Build history of the part. All positions in model axes, mm. A direction names the side the tool comes from. Coordinates: 2 decimals unless noted, no trailing zeros. Write each loop counter-clockwise with the first axis right and the second up, starting at its lowest first coordinate (ties: lowest second). Pieces come first, ordered by that corner, then holes.
```python
from build123d import *

# Parameters (mm, degrees)
SKETCH1_W           = 50
SKETCH1_H           = 110
BOSS_EXTRUDE1_DEPTH = 2
SKETCH2_W           = 50
SKETCH2_H           = 110
SKETCH2_W_2         = 46
SKETCH2_H_2         = 106
BOSS_EXTRUDE3_DEPTH = 11
SKETCH3_R           = 1.2
BOSS_EXTRUDE4_DEPTH = 11
SKETCH4_W           = 52
SKETCH4_H           = 112
SKETCH4_W_2         = 50
SKETCH4_H_2         = 110
EXTRUDE_THIN1_DEPTH = 13
FILLET2_R           = 2
EXTRUDE_THIN3_DEPTH = 3
SKETCH6_R           = 1.8
BOSS_EXTRUDE5_DEPTH = 2.8
SKETCH8_W           = 8
SKETCH8_H           = 3.6
CUT_EXTRUDE2_DEPTH  = 12.8
SKETCH11_W          = 13.1
SKETCH11_H          = 5.8
CUT_EXTRUDE5_DEPTH  = 3


with BuildPart() as part:
    # Sketch1 → Boss-Extrude1 (new body)
    with BuildSketch(Plane(origin=(0, 0, 0), x_dir=(1, 0, 0), z_dir=(0, 1, 0))):
        with Locations((-52.022587269, -1.919917864)):
            Rectangle(SKETCH1_W, SKETCH1_H)
    extrude(amount=BOSS_EXTRUDE1_DEPTH)

    # Sketch2 → Boss-Extrude3 (add)
    with BuildSketch(Plane(origin=(0, 2, 0), x_dir=(1, 0, 0), z_dir=(0, 1, 0))):
        with Locations((-52.022587269, -1.919917864)):
            Rectangle(SKETCH2_W, SKETCH2_H)
        with Locations((-52.022587269, -1.919917864)):
            Rectangle(SKETCH2_W_2, SKETCH2_H_2, mode=Mode.SUBTRACT)
    extrude(amount=BOSS_EXTRUDE3_DEPTH)

    # Sketch3 → Boss-Extrude4 (add)
    with BuildSketch(Plane(origin=(0, 2, 0), x_dir=(1, 0, 0), z_dir=(0, 1, 0))):
        with Locations((-31.022587269, 42.380082136)):
            Circle(SKETCH3_R)
        with Locations((-31.022587269, -52.919917864)):
            Circle(SKETCH3_R)
        with Locations((-56.322587269, 42.380082136)):
            Circle(SKETCH3_R)
        with Locations((-56.322587269, -52.919917864)):
            Circle(SKETCH3_R)
    extrude(amount=BOSS_EXTRUDE4_DEPTH)

    # Sketch4 → Extrude-Thin1 (add)
    with BuildSketch(Plane(origin=(0, 13, 0), x_dir=(1, 0, 0), z_dir=(0, 1, 0))):
        with Locations((-52.022587269, -1.919917864)):
            Rectangle(SKETCH4_W, SKETCH4_H)
        with Locations((-52.022587269, -1.919917864)):
            Rectangle(SKETCH4_W_2, SKETCH4_H_2, mode=Mode.SUBTRACT)
    extrude(amount=-EXTRUDE_THIN1_DEPTH)

    # Fillet2
    fillet2_edges = [part.edges().sort_by_distance(p)[0] for p in [
        (-26.022587269, 6.5, -54.080082136),
        (-26.022587269, 6.5, 57.919917864),
        (-78.022587269, 6.5, 57.919917864),
        (-78.022587269, 6.5, -54.080082136),
    ]]
    fillet(fillet2_edges, radius=FILLET2_R)

    # Sketch5 → Extrude-Thin3 (add)
    with BuildSketch(Plane(origin=(0, 13, 0), x_dir=(1, 0, 0), z_dir=(0, 1, 0))):
        with BuildLine():
            Line((-28.022587269, 54.080082136), (-76.022587269, 54.080082136))
            ThreePointArc((-76.022587269, 54.080082136), (-77.436800831, 53.494295698), (-78.022587269, 52.080082136))
            Line((-78.022587269, 52.080082136), (-78.022587269, -55.919917864))
            ThreePointArc((-78.022587269, -55.919917864), (-77.436800831, -57.334131427), (-76.022587269, -57.919917864))
            Line((-76.022587269, -57.919917864), (-28.022587269, -57.919917864))
            ThreePointArc((-28.022587269, -57.919917864), (-26.608373707, -57.334131427), (-26.022587269, -55.919917864))
            Line((-26.022587269, -55.919917864), (-26.022587269, 52.080082136))
            ThreePointArc((-26.022587269, 52.080082136), (-26.608373707, 53.494295698), (-28.022587269, 54.080082136))
        make_face()
        with BuildLine():
            Line((-28.022587269, 52.880082136), (-76.022587269, 52.880082136))
            ThreePointArc((-76.022587269, 52.880082136), (-76.588272694, 52.64576756), (-76.822587269, 52.080082136))
            Line((-76.822587269, 52.080082136), (-76.822587269, -55.919917864))
            ThreePointArc((-76.822587269, -55.919917864), (-76.588272694, -56.485603289), (-76.022587269, -56.719917864))
            Line((-76.022587269, -56.719917864), (-28.022587269, -56.719917864))
            ThreePointArc((-28.022587269, -56.719917864), (-27.456901844, -56.485603289), (-27.222587269, -55.919917864))
            Line((-27.222587269, -55.919917864), (-27.222587269, 52.080082136))
            ThreePointArc((-27.222587269, 52.080082136), (-27.456901844, 52.64576756), (-28.022587269, 52.880082136))
        make_face(mode=Mode.SUBTRACT)
    extrude(amount=EXTRUDE_THIN3_DEPTH)

    # Sketch6 → Boss-Extrude5 (add)
    with BuildSketch(Plane(origin=(0, 2, 0), x_dir=(1, 0, 0), z_dir=(0, 1, 0))):
        with Locations((-56.322587269, -52.919917864)):
            Circle(SKETCH6_R)
        with Locations((-31.022587269, -52.919917864)):
            Circle(SKETCH6_R)
        with Locations((-56.322587269, 42.380082136)):
            Circle(SKETCH6_R)
        with Locations((-31.022587269, 42.380082136)):
            Circle(SKETCH6_R)
    extrude(amount=BOSS_EXTRUDE5_DEPTH)

    # Sketch8 → Cut-Extrude2 (cut)
    with BuildSketch(Plane(origin=(-26.022587269, 0, 0), x_dir=(0, 0, -1), z_dir=(1, 0, 0))):
        with Locations((-44.619917864, 3.8)):
            Rectangle(SKETCH8_W, SKETCH8_H)
    extrude(amount=-CUT_EXTRUDE2_DEPTH, mode=Mode.SUBTRACT)

    # Sketch11 → Cut-Extrude5 (cut)
    with BuildSketch(Plane.ZY.offset(78.022587269)):
        with Locations((-43.530082136, 4.9)):
            Rectangle(SKETCH11_W, SKETCH11_H)
    extrude(amount=-CUT_EXTRUDE5_DEPTH, mode=Mode.SUBTRACT)


solid = part.part
```
1. Flat gauge pins, fed straight in: pin 1 (1.9 mm diameter, centred on x = -31.5, z = 52.5, fed in from +Y); pin 2 (2 mm diameter, centred on x = -45, z = 33, fed in from +Y). Where does each tip first touch, or does it go through?
Computed values:
pin 1: stops at y = 13
pin 2: stops at y = 2
2. Mould opens along Y. For faces 6 (the face through (-26.023, 8, 3)), 7 (the face through (-31, 13, -42)), 8 (the face through (-77, 5, -36.98)) say: +Y half, -Y half, draft (parallel to the pull), parting line (faces both ways), or undercut.
Computed values:
face 6: draft
face 7: +Y half
face 8: undercut
3. Saw through at A-A on y = 15. List the corners of the cut face in (x, z).
Computed values:
outline: (-78.02, -52.08) arc R2 ccw to (-76.02, -54.08) - (-28.02, -54.08) arc R2 ccw to (-26.02, -52.08) - (-26.02, 55.92) arc R2 ccw to (-28.02, 57.92) - (-76.02, 57.92) arc R2 ccw to (-78.02, 55.92) - close; hole (-76.82, -52.08) arc R0.8 ccw to (-76.02, -52.88) - (-28.02, -52.88) arc R0.8 ccw to (-27.22, -52.08) - (-27.22, 55.92) arc R0.8 ccw to (-28.02, 56.72) - (-76.02, 56.72) arc R0.8 ccw to (-76.82, 55.92) - close
4. Saw through at C-C on x = -70.5. List the corners of the cut face in (y, z).
Computed values:
outline: (0, -54.08) - (16, -54.08) - (16, -52.88) - (13, -52.88) - (13, -51.08) - (2, -51.08) - (2, 54.92) - (13, 54.92) - (13, 56.72) - (16, 56.72) - (16, 57.92) - (0, 57.92) - close
5. 3-axis set-ups, long thin cutter, end or side, ignore diameter. For faces 1 (the face through (-29.023, 7, 3)), 2 (the face through (-52, 0, 1)), 3 (the face through (-77, 16, 2)), 4 (the face through (-77, 7.8, -44)), 5 (the face through (-28, 5.6, 45)): which of +Z, -Z, +X, -X, +Y, -Y reach the whole face in a straight line?
Computed values:
face 1: +Y
face 2: +Z, -Z, +X, -X, -Y
face 3: +Z, -Z, +X, -X, +Y
face 4: -X
face 5: +X
6. Saw through at D-D on y = 6.75. List the corners of the cut face in (x, z), plus the area to 3 significant figures.
Computed values:
outline: (-78.02, -52.08) arc R2 ccw to (-76.02, -54.08) - (-28.02, -54.08) arc R2 ccw to (-26.02, -52.08) - (-26.02, 55.92) arc R2 ccw to (-28.02, 57.92) - (-76.02, 57.92) arc R2 ccw to (-78.02, 55.92) - (-78.02, -36.98) - (-75.02, -36.98) - (-75.02, 54.92) - (-29.02, 54.92) - (-29.02, -51.08) - (-75.02, -51.08) - (-75.02, -50.08) - (-78.02, -50.08) - close; circle Ø2.4 at (-56.32, -42.38); circle Ø2.4 at (-56.32, 52.92); circle Ø2.4 at (-31.02, -42.38); circle Ø2.4 at (-31.02, 52.92)
area: 923 mm2
7. Saw through at B-B on z = -16.5. List the corners of the cut face in (x, y), plus the area to 3 significant figures.
Computed values:
outline: (-78.02, 0) - (-26.02, 0) - (-26.02, 16) - (-27.22, 16) - (-27.22, 13) - (-29.02, 13) - (-29.02, 2) - (-75.02, 2) - (-75.02, 13) - (-76.82, 13) - (-76.82, 16) - (-78.02, 16) - close
area: 177 mm2
8. Probe line 1 along Z through (x, y) = (-44.5, 15.75); line 2 along Z through (x, y) = (-35, 10.25); line 3 along X through (y, z) = (10.75, -1). List the from-to ranges inside material, lowest first.
Computed values:
line 1: z = -54.08 to -52.88, 56.72 to 57.92
line 2: z = -54.08 to -51.08, 54.92 to 57.92
line 3: x = -78.02 to -75.02, -29.02 to -26.02
